Part model, mm, in its own coordinate system. A direction names the side the tool comes from. Give positions to 0.01 mm unless a question says otherwise; leave off trailing zeros. Write each loop counter-clockwise with the first axis right and the second up, starting at its lowest first coordinate (ties: lowest second). Pieces come first, ordered by that corner, then holes. Notation, with made-up numbers: M -18,-36.75 L 28,-36.75 A18 cw 28,-16.75 Z; hole C -30,64 d9. An arc over 180 degrees is marked long. Answer as CSV lines item,"result". Start each with the question number.
Item 1: Band-saw the part on A-A, the plane y = 4.5. List the corners of the cut face in (x, z).
Item 2: Two-plate mould, pull along Z, no slides. Class faces 1 (the flat face through (-37.5, -5, 0)), 2 (the cylindrical face through (1.802, 5.07, 5.723)), 3 (the cylindrical face through (28.945, -4.93, 28.479)): +Z half, -Z half, draft (parallel to the pull), parting line (faces both ways), or undercut.
Item 3: Pin check, flat tips, straight feed: pin 1 (10 mm diameter, centred on x = 26.5, y = 1, fed in from -Z); pin 2 (1.5 mm diameter, centred on y = -2.5, z = 9, fed in from -X); pin 3 (9.5 mm diameter, centred on x = -12.5, z = -12.5, fed in from -Y). Stop position of each tip, or through.
Item 4: Wall check: L1, parallel to X at y = -6.75, z = -12.5; L2, parallel to X at y = -5.25, z = -10; L3, parallel to Z at x = 17, y = -0.5. Give the ranges that are in metal, low to high. Write a range as from..to.
Item 5: 3-axis set-ups, long thin cutter, end or side, ignore diameter. For faces 4 (the cylindrical face through (7.177, -5.07, 9.731)), 5 (the flat face through (0, -5, -37.5)): which of +Z, -Z, +X, -X, +Y, -Y reach the whole face in a straight line?
Item 6: Band-saw the part on B-B, the plane x = 0. List the corners of the cut face in (y, z).
Item 7: Band-saw the part on C-C, the plane y = -1.25. List the corners of the cut face in (x, z).
Item 8: Band-saw the part on D-D, the plane z = 0. List the corners of the cut face in (x, y), then the cut area to 3 significant figures.
from build123d import *

# Parameters (mm, degrees)
BOSS_EXTRUDE1_DEPTH = 10
CHAMFER1_SIZE       = 10
SKETCH3_R           = 6
CUT_EXTRUDE2_DEPTH  = 10
SKETCH5_R           = 6
CUT_EXTRUDE3_DEPTH  = 10


with BuildPart() as part:
    # Sketch1 → Boss-Extrude1 (new, symmetric)
    with BuildSketch(Plane(origin=(0, 0, 0), x_dir=(1, 0, 0), z_dir=(0, 1, 0))):
        with BuildLine():
            Line((-7.5, 37.5), (7.5, 37.5))
            ThreePointArc((7.5, 37.5), (28.713203436, 28.713203436), (37.5, 7.5))
            Line((37.5, 7.5), (37.5, -7.5))
            ThreePointArc((37.5, -7.5), (28.713203436, -28.713203436), (7.5, -37.5))
            Line((7.5, -37.5), (-7.5, -37.5))
            ThreePointArc((-7.5, -37.5), (-28.713203436, -28.713203436), (-37.5, -7.5))
            Line((-37.5, -7.5), (-37.5, 7.5))
            ThreePointArc((-37.5, 7.5), (-28.713203436, 28.713203436), (-7.5, 37.5))
        make_face()
    extrude(amount=BOSS_EXTRUDE1_DEPTH, both=True)

    # Chamfer1
    chamfer1_edges = [part.edges().sort_by_distance(p)[0] for p in [
        (28.713203436, 10, 28.713203436),
        (37.5, 10, 0),
        (28.713203436, 10, -28.713203436),
        (0, 10, -37.5),
        (-28.713203436, 10, -28.713203436),
        (-37.5, 10, 0),
        (-28.713203436, 10, 28.713203436),
        (0, 10, 37.5),
    ]]
    chamfer(chamfer1_edges, length=CHAMFER1_SIZE)

    # Sketch3 → Cut-Extrude2 (cut)
    with BuildSketch(Plane.XZ.offset(10)):
        with Locations(Location((12.5, 12.5, 0), (0, 0, 270))):
            Circle(SKETCH3_R)
        with Locations(Location((-12.5, 12.5, 0), (0, 0, 270))):
            Circle(SKETCH3_R)
        with Locations(Location((12.5, -12.5, 0), (0, 0, 270))):
            Circle(SKETCH3_R)
        with Locations(Location((-12.5, -12.5, 0), (0, 0, 270))):
            Circle(SKETCH3_R)
    extrude(amount=-CUT_EXTRUDE2_DEPTH, mode=Mode.SUBTRACT)

    # Sketch5 → Cut-Extrude3 (cut)
    with BuildSketch(Plane(origin=(0, 10, 0), x_dir=(1, 0, 0), z_dir=(0, 1, 0))):
        with Locations(Location((0, 0, 0), (0, 0, 270))):
            Circle(SKETCH5_R)
    extrude(amount=-CUT_EXTRUDE3_DEPTH, mode=Mode.SUBTRACT)


solid = part.part
Output:
1,outline,"M -33,-7.5 A25.5 ccw -7.5,-33 L 7.5,-33 A25.5 ccw 33,-7.5 L 33,7.5 A25.5 ccw 7.5,33 L -7.5,33 A25.5 ccw -33,7.5 Z; hole C 0,0 d12"
2,face 1,"draft"
2,face 2,"undercut"
2,face 3,"+Z half"
3,pin 1,"z = -33.98"
3,pin 2,"x = -37.49"
3,pin 3,"y = 0"
4,L1,"-37.08..-18.5, -6.5..6.5, 18.5..37.08"
4,L2,"-37.4..-17.95, -7.05..7.05, 17.95..37.4"
4,L3,"-35.96..-16.47, -8.53..8.53, 16.47..35.96"
5,face 4,"-Y"
5,face 5,"-Z, +X, -X, +Y, -Y"
6,outline,"M -10,-37.5 L 0,-37.5 L 10,-27.5 L 10,-6 L 0,-6 L 0,6 L 10,6 L 10,27.5 L 0,37.5 L -10,37.5 Z"
7,outline,"M -37.5,-7.5 A30 ccw -7.5,-37.5 L 7.5,-37.5 A30 ccw 37.5,-7.5 L 37.5,7.5 A30 ccw 7.5,37.5 L -7.5,37.5 A30 ccw -37.5,7.5 Z; hole C -12.5,-12.5 d12; hole C -12.5,12.5 d12; hole C 12.5,-12.5 d12; hole C 12.5,12.5 d12"
8,outline,"M -37.5,-10 L 37.5,-10 L 37.5,0 L 27.5,10 L 6,10 L 6,0 L -6,0 L -6,10 L -27.5,10 L -37.5,0 Z"
8,area,"1,280 mm²"
